Here's how the part is built. I have some questions about the finished solid (model axes, mm). A direction names the side the tool comes from. Give positions to 0.01 mm unless a question says otherwise; leave off trailing zeros. Loops run counter-clockwise (first coordinate to the right, second up) from the corner with the lowest first, then second, coordinate; pieces in that order, holes last. Notation, with made-up numbers: (41.5, 8) - (74.5, 8) arc R7 cw to (74.5, 21) - close; hole circle Ø8 at (-26, 29). An arc over 180 degrees is marked (long way). Use one line per item in the form item = value.
Autodesk Inventor part; units mm, degrees
ref_plane "YZ Plane" through (0, 0, 0) normal (1, 0, 0) x (0, 1, 0)
ref_plane "XZ Plane" through (0, 0, 0) normal (0, 1, 0) x (-1, 0, 0)
ref_plane "XY Plane" through (0, 0, 0) normal (0, 0, 1) x (1, 0, 0)
sketch "Sketch1" plane through (0, 0, 0) normal (0, 0, 1) x (1, 0, 0)
  line L0 (0, 0) -> (32.5, 0)
  line L1 (32.5, 0) -> (32.5, 18.5)
  line L2 (32.5, 18.5) -> (0, 18.5)
  line L3 (0, 18.5) -> (0, 0)
  line L4 (5, 3) -> (27.5, 3)
  line L5 (27.5, 3) -> (27.5, 15.5)
  line L6 (27.5, 15.5) -> (5, 15.5)
  line L7 (5, 15.5) -> (5, 3)
  line L8 (27.5, 9.25) -> (32.5, 9.25) construction
  line L9 (5, 9.25) -> (0, 9.25) construction
  line L10 (16.25, 18.5) -> (16.25, 15.5) construction
  line L11 (16.25, 3) -> (16.25, 0) construction
  circle A0 centre (2.35, 9.25) radius 1.1
  circle A1 centre (30.15, 9.25) radius 1.1
  line L12 (32.5, 0) -> (120, 0)
  line L13 (120, 0) -> (120, 3)
  arc A2 (120, 3) -> (32.5, 18.5) centre (32.5, -236.2258) ccw
  arc A3 (116.873, 2) -> (32.5, 16.5) centre (32.5, -236.2258) ccw
  line L14 (116.873, 2) -> (32.5, 2)
  line L15 (32.5, 16.5) -> (57.6147, 2)
  line L16 (57.6147, 2) -> (76.1508, 12.7018)
  line L17 (76.1508, 12.7018) -> (94.6868, 2)
  line L18 (94.6868, 2) -> (102.617, 6.5785) construction
  line L19 (102.617, 6.5785) -> (94.6868, 2) construction
  line L20 (94.6868, 2) -> (94.1868, 2.866) construction
  line L21 (94.1868, 2.866) -> (102.117, 7.4445) construction
  line L22 (102.117, 7.4445) -> (102.617, 6.5785) construction
  line L23 (94.6868, 2) -> (76.1508, 12.7018)
  line L24 (76.1508, 12.7018) -> (76.6508, 13.5678)
  line L25 (76.6508, 13.5678) -> (96.6868, 2)
  line L26 (76.1508, 12.7018) -> (57.6147, 2)
  line L27 (57.6147, 2) -> (57.1147, 2.866)
  line L28 (57.1147, 2.866) -> (75.6508, 13.5678)
  line L29 (75.6508, 13.5678) -> (76.1508, 12.7018)
  line L30 (57.6147, 2) -> (32.5, 16.5)
  line L31 (32.5, 16.5) -> (33, 17.366)
  line L32 (33, 17.366) -> (58.1147, 2.866)
  line L33 (58.1147, 2.866) -> (57.6147, 2)
  line L34 (94.6868, 2) -> (95.1868, 1.134) construction
  line L35 (95.1868, 1.134) -> (103.117, 5.7125) construction
  line L36 (103.117, 5.7125) -> (103.9456, 6.1909) construction
  line L37 (76.1508, 12.7018) -> (75.6508, 11.8358)
  line L38 (75.6508, 11.8358) -> (92.6868, 2)
  line L39 (92.6868, 2) -> (94.6868, 2)
  line L40 (57.6147, 2) -> (58.1147, 1.134)
  line L41 (58.1147, 1.134) -> (76.6508, 11.8358)
  line L42 (76.6508, 11.8358) -> (76.1508, 12.7018)
  line L43 (32.5, 16.5) -> (32, 15.634)
  line L44 (32, 15.634) -> (57.1147, 1.134)
  line L45 (57.1147, 1.134) -> (57.6147, 2)
  line L46 (103.9456, 6.1909) -> (102.617, 6.5785)
  point P0 (32.5, 16.5)
  point P1 (101.2792, 6.9608)
  point P2 (94.6868, 3.1547)
  point P3 (79.0671, 12.1727)
  point P4 (74.6102, 12.967)
  point P5 (57.6147, 3.1547)
  point P6 (34.5139, 16.492)
  point P7 (32.5, 15.3453)
  point P8 (55.6147, 2)
  point P9 (59.6147, 2)
  point P10 (76.1508, 11.5471)
  point P11 (92.6868, 2)
  point P12 (96.6868, 2)
  dimension "d8" = 5
  dimension "d10" = 3
  dimension "d11" = 22.5
  dimension "d13" = 12.5
  dimension "d14" = 2.65
  dimension "d16" = 2.2
  dimension "d17" = 120
  dimension "d18" = 3
  dimension "d23" = 2
  dimension "d73" = 30
  dimension "d74" = 30
  dimension "d75" = 30
  dimension "d76" = 30
  dimension "d77" = 1
extrude "Extrusion1" add sketch "Sketch1" along normal mid plane 5 contours L3 L2 L1 L43 L44 L0 | L1 L14 L44 L45 L40 L41 A3 L25 L24 L29 L28 L32 L31 A2 L13 L12 | L44 L43 L1 | L1 L15 L14 L44 | L14 L45 L44 | L31 L32 A3 | A3 L32 L28 L27 L15 | L16 L37 L38 L41 L14 | L33 L32 L28 A3 L16 | L27 L28 L32 L33 | L14 L41 L40 | L24 L25 A3 | A3 L25 L14 L17 | A3 L28 L29 | L42 L41 L38 L37 | L17 L14 L38 L41 L42
fillet "Fillet3" radius 2 4 edges at (0, 18.5, 0) (0, 0, 0) (120, 0, 0) (120, 3, 0)
fillet "Fillet5" radius 3 5 edges at (76.1508, 11.5471, 0) (32.5, 15.3453, 0) (57.6147, 3.1547, 0) (96.6868, 2, 0) (32.5, 2, 0)
fillet "Fillet5" radius 1 7 edges at (116.873, 2, 0) (92.6868, 2, 0) (79.0671, 12.1727, 0) (34.5139, 16.492, 0) (74.6102, 12.967, 0) (59.6147, 2, 0) (55.6147, 2, 0)
properties part number "foot_v0.1"
(1) For P1, Ø2.5, axis at x = 40, z = 0, coming from the +Y side, with a flat end and sliding along its axis, tell me the tip position at first contact or that it passes through.
Geometry says:
P1 = 18.42
(2) Thinking about a two-plate mould opening in X: for faces 1 (the flat face through (5, 9, 0)), 2 (the flat face through (17, 18.5, 0)), which applies, pulls with the +X half, pulls with the -X half, needs draft (parallel to the pull), parting line crosses it, or undercut?
Geometry says:
face_1 = undercut
face_2 = needs draft
(3) If we section it at C-C (z = 0.4): Give the number of separate pieces and of enclosed holes in the cut face, plus the area to 3 significant figures.
Geometry says:
separate_pieces = 1
enclosed_holes = 7
area = 825 mm²
(4) If I drill on probe 1 along Y at (x, z) = (2.35, -0.4); probe 2 along Y at (x, z) = (20, -1.9); probe 3 along Y at (x, z) = (67, -0.3), over which ranges is the centre line in solid material (lowest first)?
Geometry says:
probe_1 = 0 to 8.15, 10.35 to 18.5
probe_2 = 0 to 3, 15.5 to 18.5
probe_3 = 0 to 2, 6.26 to 8.57, 14.13 to 16.15
(5) For faces 3 (the cylindrical face through (76.173, 11.083, 0.035)), 4 (the flat face through (45, 9, -2.5)), which set-ups out of +Z, -Z, +X, -X, +Y, -Y let a thin tool reach every point of the face, with its end or its side?
Geometry says:
face_3 = +Z, -Z
face_4 = -Z, +X, -X, +Y, -Y
(6) If we section it at A-A (x = 26): List the corners of the cut face in (y, z) for me.
Geometry says:
outline = (0, -2.5) - (3, -2.5) - (3, 2.5) - (0, 2.5) - close; (15.5, -2.5) - (18.5, -2.5) - (18.5, 2.5) - (15.5, 2.5) - close
(7) If we section it at B-B (x = 68): List the corners of the cut face in (y, z) for me, plus the area to 3 significant figures.
Geometry says:
outline = (0, -2.5) - (2, -2.5) - (2, 2.5) - (0, 2.5) - close; (6.84, -2.5) - (9.15, -2.5) - (9.15, 2.5) - (6.84, 2.5) - close; (13.99, -2.5) - (16.01, -2.5) - (16.01, 2.5) - (13.99, 2.5) - close
area = 31.6 mm²
